CAD build for the part. Positions are in the model's coordinates, mm. A direction names the side the tool comes from. Coordinates: 2 decimals unless noted, no trailing zeros. Loops run counter-clockwise (first coordinate to the right, second up) from the corner with the lowest first, then second, coordinate; pieces in that order, holes last. Notation, with made-up numbers: (28, 63.5) -> (64, 63.5) arc R21 cw to (64, 85.5) -> close; hole circle Ø5 at (87.25, 88). An arc over 180 degrees is marked (long way). Write each question's results on one line, items separated by ' | '.
from build123d import *

# Parameters (mm, degrees)
F0_R     = 17.5
F1_DEPTH = 76
F2_DEPTH = 7
F3_R     = 2


with BuildPart() as f1:
    # F0 (on Front) → F1 (new body)
    with BuildSketch(Plane.XZ):
        with BuildLine():
            Line((23.5, 25.5), (-23.5, 25.5))
            ThreePointArc((-23.5, 25.5), (-24.9142135624, 24.9142135624), (-25.5, 23.5))
            Line((-25.5, 23.5), (-25.5, -23.5))
            ThreePointArc((-25.5, -23.5), (-24.9142135624, -24.9142135624), (-23.5, -25.5))
            Line((-23.5, -25.5), (23.5, -25.5))
            ThreePointArc((23.5, -25.5), (24.9142135624, -24.9142135624), (25.5, -23.5))
            Line((25.5, -23.5), (25.5, 23.5))
            ThreePointArc((25.5, 23.5), (24.9142135624, 24.9142135624), (23.5, 25.5))
        make_face()
        Circle(F0_R, mode=Mode.SUBTRACT)
        Circle(F0_R)
    extrude(amount=F1_DEPTH)

    # F0 (on Front) → F2 (join)
    with BuildSketch(Plane.XZ):
        Circle(F0_R)
    extrude(amount=-F2_DEPTH)

    # F3
    f3_edges = [f1.edges().sort_by_distance(p)[0] for p in [
        (25.5, -76, 0),
    ]]
    fillet(f3_edges, radius=F3_R)


solid = f1.part
1) Pin check, flat tip, straight feed: pin 1 (4 mm diameter, centred on x = -13, z = 16, fed in from +Y). Stop position of the tip, or through.
Outcome:
pin 1: stops at y = 0
2) Slice it at A-A (z = 0). Write the cut outline in (x, y), then the cut area to 3 significant figures.
Outcome:
outline: (-25.5, -74) arc R2 ccw to (-23.5, -76) -> (23.5, -76) arc R2 ccw to (25.5, -74) -> (25.5, 0) -> (17.5, 0) -> (17.5, 7) -> (-17.5, 7) -> (-17.5, 0) -> (-25.5, 0) -> close | area: 4,120 mm^2
3) Slice it at C-C (z = -20). Write the cut outline in (x, y).
Outcome:
outline: (-25.5, -74) arc R2 ccw to (-23.5, -76) -> (23.5, -76) arc R2 ccw to (25.5, -74) -> (25.5, 0) -> (-25.5, 0) -> close
4) Slice it at B-B (x = 0). Write the cut outline in (y, z), then the cut area to 3 significant figures.
Outcome:
outline: (-76, -23.5) arc R2 ccw to (-74, -25.5) -> (0, -25.5) -> (0, -17.5) -> (7, -17.5) -> (7, 17.5) -> (0, 17.5) -> (0, 25.5) -> (-74, 25.5) arc R2 ccw to (-76, 23.5) -> close | area: 4,120 mm^2
5) Slice it at D-D (x = -18.5). Write the cut outline in (y, z), then the cut area to 3 significant figures.
Outcome:
outline: (-76, -23.5) arc R2 ccw to (-74, -25.5) -> (0, -25.5) -> (0, 25.5) -> (-74, 25.5) arc R2 ccw to (-76, 23.5) -> close | area: 3,870 mm^2
6) Which spindle directions (+Z, -Z, +X, -X, +Y, -Y) get a long thin tool onto all of the face, cutting with end or side? Do faces 1 (the cylindrical face through (-13.887, 3.451, -10.648)), 2 (the cylindrical face through (-0.33, -75.43, 24.9)). Say none if no direction does.
Outcome:
face 1: +Y | face 2: +Z, +X, -X, -Y
7) Drill centre lines: L1, parallel to Y at x = -19, z = 15.5; L2, parallel to X at y = 2, z = 15. Where is each one in solid material? Low to high. Write a range as from..to.
Outcome:
L1: y = -76..0 | L2: x = -9.01..9.01
